Read the model definition and answer for the solid it produces. Units are mm, in the model's axes. Face numbers are marked on the shaded views. Coordinates: 2 decimals unless noted, no trailing zeros. Loops run counter-clockwise (first coordinate to the right, second up) from the corner with the lowest first, then second, coordinate; pieces in that order, holes last. Notation, with made-up numbers: M 38.25,2.25 L 50.25,2.25 A23 cw 50.25,37.25 Z; hole C -4.5,-20.75 d4. An arc over 180 degrees is marked long. Put each result on its own line as item: value.
from build123d import *

# Parameters (mm, degrees)
SKETCH3_W           = 18.499327609
SKETCH3_H           = 18.499327609
BOSS_EXTRUDE2_DEPTH = 12.7
FILLET2_R           = 2.54
SKETCH4_R           = 6.35
SKETCH4_R_2         = 1.778
CUT_EXTRUDE1_DEPTH  = 12.7


with BuildPart() as part:
    # Sketch3 → Boss-Extrude2 (new body)
    with BuildSketch(Plane(origin=(0, 0, 0), x_dir=(1, 0, 0), z_dir=(0, 1, 0))):
        with Locations((-9.249663805, 9.249663805)):
            Rectangle(SKETCH3_W, SKETCH3_H)
    extrude(amount=BOSS_EXTRUDE2_DEPTH)

    # Fillet2
    fillet2_edges = [part.edges().sort_by_distance(p)[0] for p in [
        (0, 6.35, 0),
        (-18.499327609, 6.35, 0),
        (-18.499327609, 6.35, -18.499327609),
        (0, 6.35, -18.499327609),
    ]]
    fillet(fillet2_edges, radius=FILLET2_R)

    # Sketch4 → Cut-Extrude1 (cut)
    with BuildSketch(Plane(origin=(0, 12.7, 0), x_dir=(1, 0, 0), z_dir=(0, 1, 0))):
        with Locations(Location((-9.249663805, 9.249663805, 0), (0, 0, 270))):
            Circle(SKETCH4_R)
        with Locations(Location((-2.334866591, 2.334866591, 0), (0, 0, 270))):
            Circle(SKETCH4_R_2)
        with Locations(Location((-16.164461018, 2.334866591, 0), (0, 0, 270))):
            Circle(SKETCH4_R_2)
        with Locations(Location((-16.164461018, 16.164461018, 0), (0, 0, 270))):
            Circle(SKETCH4_R_2)
        with Locations(Location((-2.334866591, 16.164461018, 0), (0, 0, 270))):
            Circle(SKETCH4_R_2)
    extrude(amount=-CUT_EXTRUDE1_DEPTH, mode=Mode.SUBTRACT)


solid = part.part
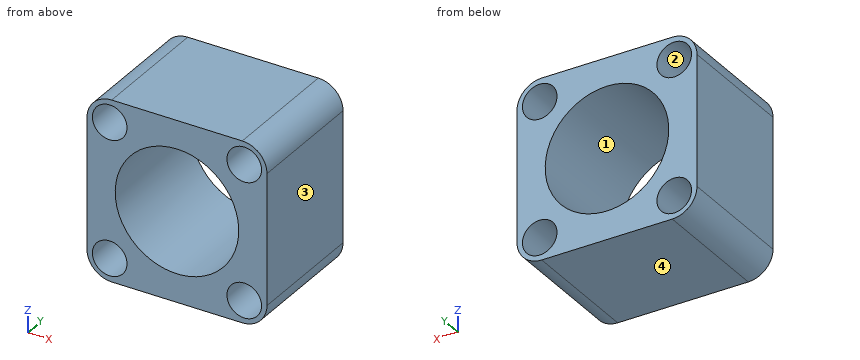
1) Find section B-B, the plane z = -3.5. Write down the section's boundary in (x, y).
Answer list:
outline: M -18.5,0 L -17.51,0 L -17.51,12.7 L -18.5,12.7 Z; M -14.82,0 L -11.94,0 L -11.94,12.7 L -14.82,12.7 Z; M -6.55,0 L -3.68,0 L -3.68,12.7 L -6.55,12.7 Z; M -0.99,0 L 0,0 L 0,12.7 L -0.99,12.7 Z
2) Given pin 1 Ø3 at (x, z) = (-16.16, -16.16) entering from +Y; pin 2 Ø4 at (x, z) = (-7, -3.5) entering from -Y, each flat-ended and moving along its own axis, determine where each tip first touches the part or whether it passes through.
Answer list:
pin 1: passes through
pin 2: stops at y = 0
3) Straight lines are drawn through the part: line 1 (Z direction, x = -9.25, y = 9.75); line 2 (Z direction, x = -17.5, y = 9.5). For each, find the intervals that lie inside material, in ascending order. Write a range as [from, to].
Answer list:
line 1: z = [-18.5, -15.6], [-2.9, 0]
line 2: z = [-17.98, -17.34], [-14.99, -3.51], [-1.16, -0.52]
4) Find section D-D, the plane y = 3.75. Write down the section's boundary in (x, z), plus the area to 3 significant figures.
Answer list:
outline: M -18.5,-15.96 A2.54 ccw -15.96,-18.5 L -2.54,-18.5 A2.54 ccw 0,-15.96 L 0,-2.54 A2.54 ccw -2.54,0 L -15.96,0 A2.54 ccw -18.5,-2.54 Z; hole C -16.16,-16.16 d3.56; hole C -16.16,-2.33 d3.56; hole C -9.25,-9.25 d12.7; hole C -2.33,-16.16 d3.56; hole C -2.33,-2.33 d3.56
area: 170 mm^2
5) Determine the mould class of the marked faces 1, 2, 3 and 4 for opening direction X: released by +X, released by -X, zero draft, split by the parting line, or undercut.
Answer list:
face 1: undercut
face 2: undercut
face 3: released by +X
face 4: zero draft
6) Find section A-A, the plane x = -5. Write down the section's boundary in (y, z).
Answer list:
outline: M 0,-18.5 L 12.7,-18.5 L 12.7,-13.97 L 0,-13.97 Z; M 0,-4.53 L 12.7,-4.53 L 12.7,0 L 0,0 Z
7) Find section C-C, the plane x = -2. Write down the section's boundary in (y, z).
Answer list:
outline: M 0,-18.44 L 12.7,-18.44 L 12.7,-17.91 L 0,-17.91 Z; M 0,-14.42 L 12.7,-14.42 L 12.7,-4.08 L 0,-4.08 Z; M 0,-0.59 L 12.7,-0.59 L 12.7,-0.06 L 0,-0.06 Z
